```python
from build123d import *

# Parameters (mm, degrees)
SKETCH2_W           = 29.75
SKETCH2_H           = 36.25
BOSS_EXTRUDE1_DEPTH = 33.75
SKETCH3_R           = 14.3
BOSS_EXTRUDE2_DEPTH = 7
SKETCH4_R           = 10.875
BOSS_EXTRUDE3_DEPTH = 5.5
SKETCH5_R           = 13.5
BOSS_EXTRUDE4_DEPTH = 13.95
SKETCH6_R           = 19.8
BOSS_EXTRUDE5_DEPTH = 4.3
SKETCH7_W           = 23.2
SKETCH7_H           = 10
BOSS_EXTRUDE6_DEPTH = 1


with BuildPart() as part:
    # Sketch2 → Boss-Extrude1 (new body)
    with BuildSketch(Plane(origin=(0, 0, 0), x_dir=(1, 0, 0), z_dir=(0, 1, 0))):
        Rectangle(SKETCH2_W, SKETCH2_H)
    extrude(amount=BOSS_EXTRUDE1_DEPTH)

    # Sketch3 → Boss-Extrude2 (add)
    with BuildSketch(Plane(origin=(0, 33.75, 0), x_dir=(1, 0, 0), z_dir=(0, 1, 0))):
        Circle(SKETCH3_R)
    extrude(amount=BOSS_EXTRUDE2_DEPTH)

    # Sketch4 → Boss-Extrude3 (add)
    with BuildSketch(Plane(origin=(0, 40.75, 0), x_dir=(1, 0, 0), z_dir=(0, 1, 0))):
        Circle(SKETCH4_R)
    extrude(amount=BOSS_EXTRUDE3_DEPTH)

    # Sketch5 → Boss-Extrude4 (add)
    with BuildSketch(Plane(origin=(0, 46.25, 0), x_dir=(1, 0, 0), z_dir=(0, 1, 0))):
        Circle(SKETCH5_R)
    extrude(amount=BOSS_EXTRUDE4_DEPTH)

    # Sketch6 → Boss-Extrude5 (add)
    with BuildSketch(Plane(origin=(0, 60.2, 0), x_dir=(1, 0, 0), z_dir=(0, 1, 0))):
        Circle(SKETCH6_R)
    extrude(amount=BOSS_EXTRUDE5_DEPTH)

    # Sketch7 → Boss-Extrude6 (add)
    with BuildSketch(Plane(origin=(14.875, 0, 0), x_dir=(0, 0, -1), z_dir=(1, 0, 0))):
        with Locations((0, 5)):
            Rectangle(SKETCH7_W, SKETCH7_H)
    extrude(amount=BOSS_EXTRUDE6_DEPTH)


solid = part.part
```
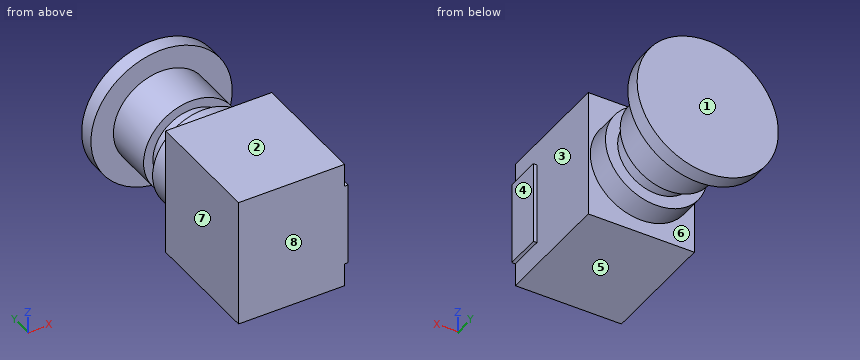
The model under review builds one solid part; all positions refer to its coordinate system, in mm. Face numbers are marked on the shaded views. A direction names the side the tool comes from. Coordinates: 2 decimals unless noted, no trailing zeros. Order: outer loops, then holes, each group sorted by start corner. A loop starts at its lowest first (then second) coordinate and runs counter-clockwise, first axis right, second up. Notation, with made-up numbers: (19.5, 41) -> (27.5, 41) arc R16 ccw to (27.5, 53) -> close; hole circle Ø7 at (-5.75, -3.5). An arc over 180 degrees is marked (long way). Answer in a Markdown table with one row per item. Add a question column.
Item 1: To check wall thickness, follow probe 1 along Y at (x, z) = (8, -14); probe 2 along Y at (x, z) = (-8.5, -7.5); probe 3 along X at (y, z) = (9, -15.5) (3 decimals). State the ranges of each line that lie inside material, in increasing order.
Item 2: Machinability: for the marked faces 4, 5, 6, 7 and 8, which of the approach directions +Z, -Z, +X, -X, +Y, -Y give a long, thin tool a straight path to every point of the face, cutting with its end or side? Answer none if there is none.
Item 3: We need section B-B on x = 12. Write out the cut boundary in (y, z) (3 decimals).
Item 4: We need section D-D on y = 14. Write out the cut boundary in (x, z) (3 decimals).
Item 5: We need section A-A on z = 0. Write out the cut boundary in (x, y) (3 decimals).
Item 6: We need section C-C on x = 0. Write out the cut boundary in (y, z) (3 decimals), plus the area to 3 significant figures.
Item 7: Clearance check with flat-ended pins moving along their axes: pin 1 (5 mm diameter, centred on x = 10, y = 32.5, fed in from -Z) (3 decimals); pin 2 (1.1 mm diameter, centred on x = 15.5, y = 3.5, fed in from +Z); pin 3 (1.1 mm diameter, centred on x = 15.5, y = 3.5, fed in from -Z). State where each tip first meets the part, or that it passes through.
Item 8: Mouldability with a two-part tool opening along Y and no side actions: class the marked faces 1, 2 and 3 as +Y half, -Y half, draft (parallel to the pull), parting line (faces both ways), or undercut.
Final values:
| question | item | result |
|---|---|---|
| 1 | probe 1 | y = 0 to 33.75, 60.2 to 64.5 |
| 1 | probe 2 | y = 0 to 40.75, 46.25 to 64.5 |
| 1 | probe 3 | x = -14.875 to 14.875 |
| 2 | face 4 | +Z, -Z, +X, -Y |
| 2 | face 5 | -Z, +X, -X, -Y |
| 2 | face 6 | none |
| 2 | face 7 | +Z, -Z, -X, -Y |
| 2 | face 8 | +Z, -Z, +X, -X, -Y |
| 3 | outline | (0, -18.125) -> (33.75, -18.125) -> (33.75, -7.778) -> (40.75, -7.778) -> (40.75, 7.778) -> (33.75, 7.778) -> (33.75, 18.125) -> (0, 18.125) -> close; (46.25, -6.185) -> (60.2, -6.185) -> (60.2, -15.749) -> (64.5, -15.749) -> (64.5, 15.749) -> (60.2, 15.749) -> (60.2, 6.185) -> (46.25, 6.185) -> close |
| 4 | outline | (-14.875, -18.125) -> (14.875, -18.125) -> (14.875, 18.125) -> (-14.875, 18.125) -> close |
| 5 | outline | (-19.8, 60.2) -> (-13.5, 60.2) -> (-13.5, 46.25) -> (-10.875, 46.25) -> (-10.875, 40.75) -> (-14.3, 40.75) -> (-14.3, 33.75) -> (-14.875, 33.75) -> (-14.875, 0) -> (15.875, 0) -> (15.875, 10) -> (14.875, 10) -> (14.875, 33.75) -> (14.3, 33.75) -> (14.3, 40.75) -> (10.875, 40.75) -> (10.875, 46.25) -> (13.5, 46.25) -> (13.5, 60.2) -> (19.8, 60.2) -> (19.8, 64.5) -> (-19.8, 64.5) -> close |
| 6 | outline | (0, -18.125) -> (33.75, -18.125) -> (33.75, -14.3) -> (40.75, -14.3) -> (40.75, -10.875) -> (46.25, -10.875) -> (46.25, -13.5) -> (60.2, -13.5) -> (60.2, -19.8) -> (64.5, -19.8) -> (64.5, 19.8) -> (60.2, 19.8) -> (60.2, 13.5) -> (46.25, 13.5) -> (46.25, 10.875) -> (40.75, 10.875) -> (40.75, 14.3) -> (33.75, 14.3) -> (33.75, 18.125) -> (0, 18.125) -> close |
| 6 | area | 2,090 mm2 |
| 7 | pin 1 | stops at z = -18.125 |
| 7 | pin 2 | stops at z = 11.6 |
| 7 | pin 3 | stops at z = -11.6 |
| 8 | face 1 | +Y half |
| 8 | face 2 | draft |
| 8 | face 3 | undercut |
